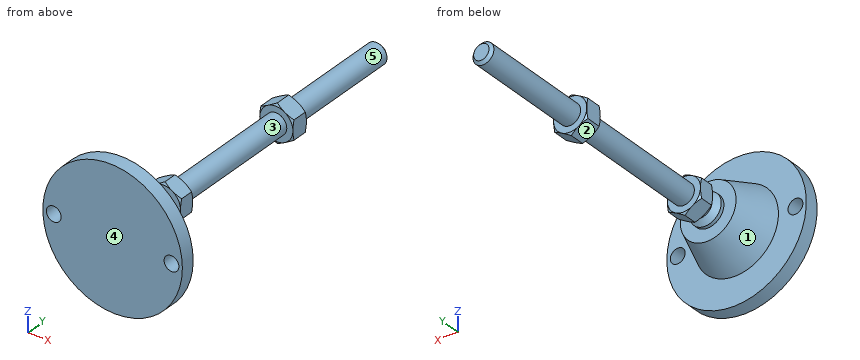
```python
from build123d import *

# Parameters (mm, degrees)
EXTRUDE_1_DEPTH     = 9
EXTRUDE_2_DEPTH     = 10
SKETCH_5_R          = 4.25
CUT_EXTRUDE_1_DEPTH = 9


with BuildPart() as part:
    # Эскиз1 → Повернуть1 (revolve)
    with BuildSketch(Plane.XY, mode=Mode.PRIVATE) as revolve_1_sk:
        Polygon((0, 0), (-40, 0), (-40, 8), (-24, 8), (-16, 29), (-9, 29), (-9, 31), (-6, 34), (-6, 38), (-6, 47), (-6, 195.4), (-4.4, 197), (0, 197), align=None)
    revolve(revolve_1_sk.sketch.rotate(Axis((0, 0, 0), (0, 1, 0)), 180), axis=Axis((0, 0, 0), (0, 1, 0)))  # turned: the seam where the file's is

    # Эскиз2 → Бобышка-Вытянуть1 (add)
    with BuildSketch(Plane(origin=(0, 38, 0), x_dir=(1, 0, 0), z_dir=(0, 1, 0))):
        Polygon((0, 10.969655115), (-9.5, 5.484827557), (-9.5, -5.484827557), (0, -10.969655115), (9.5, -5.484827557), (9.5, 5.484827557), align=None)
    extrude(amount=EXTRUDE_1_DEPTH)

    # Эскиз3 → Бобышка-Вытянуть2 (add)
    with BuildSketch(Plane(origin=(0, 121.2, 0), x_dir=(1, 0, 0), z_dir=(0, 1, 0))):
        Polygon((9.5, 5.484827557), (0, 10.969655115), (-9.5, 5.484827557), (-9.5, -5.484827557), (0, -10.969655115), (9.5, -5.484827557), align=None)
    extrude(amount=EXTRUDE_2_DEPTH)

    # Эскиз4 → Вырез-Повернуть2 (revolve, cut)
    with BuildSketch(Plane.XY, mode=Mode.PRIVATE) as cut_revolve_2_sk:
        Polygon((-18.160254038, 131.2), (-9.5, 131.2), (-18.160254038, 126.2), align=None)
        Polygon((-18.160254038, 121.2), (-18.160254038, 126.2), (-9.5, 121.2), align=None)
        Polygon((-17.294228634, 47), (-17.294228634, 42.5), (-9.5, 47), align=None)
        Polygon((-17.294228634, 42.5), (-17.294228634, 38), (-9.5, 38), align=None)
    revolve(cut_revolve_2_sk.sketch.rotate(Axis((0, 197, 0), (0, -1, 0)), 180), axis=Axis((0, 197, 0), (0, -1, 0)), mode=Mode.SUBTRACT)  # turned: the seam where the file's is

    # Эскиз5 → Вырез-Вытянуть1 (cut, through all)
    with BuildSketch(Plane(origin=(0, 8, 0), x_dir=(1, 0, 0), z_dir=(0, 1, 0))):
        with Locations(Location((-33.75, 0, 0), (0, 0, 180))):  # turned: the seam where the file's is
            Circle(SKETCH_5_R)
        with Locations(Location((33.75, 0, 0), (0, 0, 180))):  # turned: the seam where the file's is
            Circle(SKETCH_5_R)
    extrude(amount=-CUT_EXTRUDE_1_DEPTH, mode=Mode.SUBTRACT)


solid = part.part
```
Can you work these out from the model? Positions are in its coordinate system, mm. Face numbers are marked on the shaded views. A direction names the side the tool comes from. Give positions to 0.01 mm unless a question says otherwise; leave off trailing zeros. Loops run counter-clockwise (first coordinate to the right, second up) from the corner with the lowest first, then second, coordinate; pieces in that order, holes last. Notation, with made-up numbers: M 57,-25.75 L 97,-25.75 A13 cw 97,-18.75 Z; hole C -14.75,-30.5 d4. An arc over 180 degrees is marked long. One line per item, written item: value.
(1) Suppose I cut it at C-C on y = 70. List the corners of the cut face in (x, z) for me.
Returned:
outline: C 0,0 d12
(2) We'd pull the mould along Y, two halves only. Please class the marked faces 1, 2 and 3: released by +Y, released by -Y, zero draft, split by the parting line, or undercut.
Returned:
face 1: released by +Y
face 2: zero draft
face 3: undercut
(3) Will these pins go through, and if not, where does the flat tip stop? pin 1 (8 mm diameter, centred on y = 79, z = 1.5, fed in from +X); pin 2 (8 mm diameter, centred on y = 125.5, z = -1.5, fed in from +X); pin 3 (6 mm diameter, centred on x = -27.5, z = -1.5, fed in from +Y); pin 4 (7 mm diameter, centred on x = 33.75, z = 0, fed in from -Y).
Returned:
pin 1: x = 6
pin 2: x = 9.5
pin 3: y = 8
pin 4: through
(4) Suppose I cut it at D-D on z = 27. List the corners of the cut face in (x, y) for me, plus the area to 3 significant figures.
Returned:
outline: M -29.51,0 L 29.51,0 L 29.51,8 L -29.51,8 Z
area: 472 mm^2
(5) Suppose I cut it at A-A on x = 33.75. List the corners of the cut face in (y, z) for me, plus the area to 3 significant figures.
Returned:
outline: M 0,-21.47 L 8,-21.47 L 8,-4.25 L 0,-4.25 Z; M 0,4.25 L 8,4.25 L 8,21.47 L 0,21.47 Z
area: 276 mm^2
(6) I need wall thicknesses on line 1 (Y direction, x = 12.5, z = 29); line 2 (Y direction, x = -9.5, z = 10); line 3 (Z direction, x = -33, y = 3). Which ranges of each line are inside material? Lowest first, please.
Returned:
line 1: 0 to 8
line 2: 0 to 29
line 3: -22.61 to -4.18, 4.18 to 22.61
(7) Which directions (+Z, -Z, +X, -X, +Y, -Y) give clear straight access to the entire face, cutting with the end or side of a thin tool? Please do the marked faces 4 and 5.
Returned:
face 4: +Z, -Z, +X, -X, -Y
face 5: +Y
(8) Suppose I cut it at B-B on y = 41. List the corners of the cut face in (x, z) for me.
Returned:
outline: M -9.5,-5.48 L 0,-10.97 L 9.5,-5.48 L 9.5,5.48 L 0,10.97 L -9.5,5.48 Z
